Part model, mm, in its own coordinate system. A direction names the side the tool comes from. Coordinates: 2 decimals unless noted, no trailing zeros. Loops run counter-clockwise (first coordinate to the right, second up) from the corner with the lowest first, then second, coordinate; pieces in that order, holes last. Notation, with made-up numbers: M 79,38.25 L 89,38.25 A15 cw 89,55.25 Z; hole C -18,-13.5 d4. An arc over 180 degrees is marked long. Answer as a JSON object with one key per item and string values. Group by question number.
1. Saw through at A-A on x = 0. Write the cut outline in (y, z).
2. Saw through at B-B on y = 8. Write the cut outline in (x, z).
3. Drill centre lines: L1, parallel to X at y = 5.75, z = 15.5; L2, parallel to X at y = 16.25, z = 0; L3, parallel to Z at x = -16, y = 5. Where is each one in solid material? Low to high.
4. Mould opens along X. For faces 1 (the face through (-24.5, -16, 0)), 2 (the face through (3.755, 7.605, 11.923)), 3 (the face through (21, -53, 0)) say: released by +X, released by -X, zero draft, split by the parting line, or undercut.
5. 3-axis set-ups, long thin cutter, end or side, ignore diameter. For faces 4 (the face through (-10.648, 17.535, -13.887)), 5 (the face through (-21, -53, 0)), 6 (the face through (11, 0, -8)): which of +Z, -Z, +X, -X, +Y, -Y reach the whole face in a straight line?
6. Saw through at D-D on x = -15.5. Write the cut outline in (y, z).
7. Saw through at C-C on z = 15.5. Write the cut outline in (x, y).
8. Drop flat-ended pins along their axis: pin 1 Ø1.5 at (x, z) = (-9, -9.5) entering from -Y; pin 2 Ø4 at (x, z) = (-15.5, 15.5) entering from +Y; pin 3 Ø17.5 at (x, z) = (0, 4.5) entering from +Y. Give the stop position or say it passes through.
from build123d import *

# Parameters (mm, degrees)
SKETCH1_W           = 49
SKETCH1_H           = 70
BOSS_EXTRUDE1_DEPTH = 20
SKETCH3_R           = 12.5
CUT_EXTRUDE1_DEPTH  = 70
SKETCH4_R           = 1.5
CUT_EXTRUDE2_DEPTH  = 48.172555581
SKETCH5_R           = 17.5
SKETCH5_R_2         = 12.5
CUT_EXTRUDE3_DEPTH  = 5
SKETCH6_W           = 7
SKETCH6_H           = 70
BOSS_EXTRUDE3_DEPTH = 53


with BuildPart() as part:
    # Sketch1 → Boss-Extrude1 (new body)
    with BuildSketch(Plane(origin=(0, 0, 0), x_dir=(1, 0, 0), z_dir=(0, 1, 0))):
        Rectangle(SKETCH1_W, SKETCH1_H)
    extrude(amount=BOSS_EXTRUDE1_DEPTH)

    # Sketch3 → Cut-Extrude1 (cut)
    with BuildSketch(Plane(origin=(0, 20, 0), x_dir=(1, 0, 0), z_dir=(0, 1, 0))):
        with Locations(Location((0, 0, 0), (0, 0, 270))):
            Circle(SKETCH3_R)
    extrude(amount=-CUT_EXTRUDE1_DEPTH, mode=Mode.SUBTRACT)

    # Sketch4 → Cut-Extrude2 (cut, through all)
    with BuildSketch(Plane.XZ):
        with Locations(Location((-15.5, 15.5, 0), (0, 0, 270))):
            Circle(SKETCH4_R)
        with Locations(Location((15.5, 15.5, 0), (0, 0, 270))):
            Circle(SKETCH4_R)
        with Locations(Location((15.5, -15.5, 0), (0, 0, 270))):
            Circle(SKETCH4_R)
        with Locations(Location((-15.5, -15.5, 0), (0, 0, 270))):
            Circle(SKETCH4_R)
    extrude(amount=-CUT_EXTRUDE2_DEPTH, mode=Mode.SUBTRACT)

    # Sketch5 → Cut-Extrude3 (cut)
    with BuildSketch(Plane(origin=(0, 20, 0), x_dir=(1, 0, 0), z_dir=(0, 1, 0))):
        with Locations(Location((0, 0, 0), (0, 0, 270))):
            Circle(SKETCH5_R)
        with Locations(Location((0, 0, 0), (0, 0, 270))):
            Circle(SKETCH5_R_2, mode=Mode.SUBTRACT)
    extrude(amount=-CUT_EXTRUDE3_DEPTH, mode=Mode.SUBTRACT)

    # Sketch6 → Boss-Extrude3 (add)
    with BuildSketch(Plane.XZ):
        with Locations((-21, 0)):
            Rectangle(SKETCH6_W, SKETCH6_H)
        with Locations((21, 0)):
            Rectangle(SKETCH6_W, SKETCH6_H)
    extrude(amount=BOSS_EXTRUDE3_DEPTH)


solid = part.part
Outcome:
{
 "1": {"outline": "M 0,-35 L 20,-35 L 20,-17.5 L 15,-17.5 L 15,-12.5 L 0,-12.5 Z; M 0,12.5 L 15,12.5 L 15,17.5 L 20,17.5 L 20,35 L 0,35 Z"},
 "2": {"outline": "M -24.5,-35 L 24.5,-35 L 24.5,35 L -24.5,35 Z; hole C -15.5,-15.5 d3; hole C -15.5,15.5 d3; hole C 0,0 d25; hole C 15.5,-15.5 d3; hole C 15.5,15.5 d3"},
 "3": {"L1": "x = -24.5 to -17, -14 to 14, 17 to 24.5", "L2": "x = -24.5 to -17.5, 17.5 to 24.5", "L3": "z = -35 to -16.91, -14.09 to 14.09, 16.91 to 35"},
 "4": {"face 1": "released by -X", "face 2": "undercut", "face 3": "zero draft"},
 "5": {"face 4": "+Y", "face 5": "+Z, -Z, +X, -X, -Y", "face 6": "+Z, -Z, -Y"},
 "6": {"outline": "M 0,-35 L 20,-35 L 20,-17 L 0,-17 Z; M 0,-14 L 20,-14 L 20,-8.12 L 15,-8.12 L 15,8.12 L 20,8.12 L 20,14 L 0,14 Z; M 0,17 L 20,17 L 20,35 L 0,35 Z"},
 "7": {"outline": "M -24.5,-53 L -17.5,-53 L -17.5,0 L -17,0 L -17,20 L -24.5,20 Z; M -14,0 L 14,0 L 14,20 L 8.12,20 L 8.12,15 L -8.12,15 L -8.12,20 L -14,20 Z; M 17,0 L 17.5,0 L 17.5,-53 L 24.5,-53 L 24.5,20 L 17,20 Z"},
 "8": {"pin 1": "stops at y = 0", "pin 2": "stops at y = 20", "pin 3": "stops at y = 15"}
}
